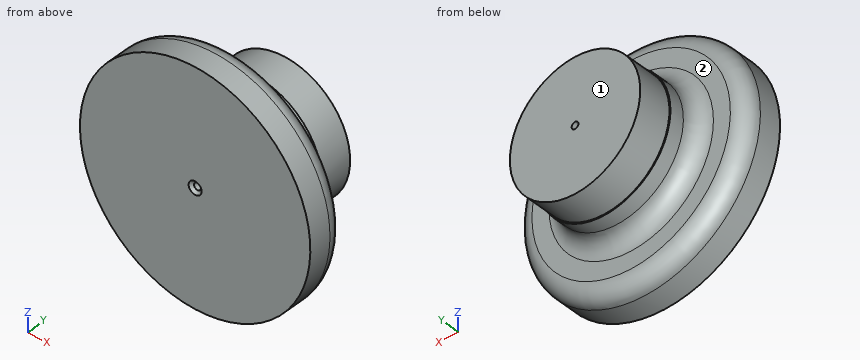
from build123d import *

# Parameters (mm, degrees)
SKETCH1_R                                           = 114.3
SKETCH1_R_2                                         = 65.7225
BOSS_EXTRUDE1_DEPTH                                 = 38.1
SKETCH1_3_R                                         = 65.7225
SKETCH1_3_R_2                                       = 64.7065
BOSS_EXTRUDE2_DEPTH                                 = 68.58
SKETCH1_4_R                                         = 64.7065
BOSS_EXTRUDE3_DEPTH                                 = 101.6
CSK_FOR_1_4_FLAT_HEAD_MACHINE_SCREW_100_D           = 6.7564
CSK_FOR_1_4_FLAT_HEAD_MACHINE_SCREW_100_CSINK_D     = 12.8778
CSK_FOR_1_4_FLAT_HEAD_MACHINE_SCREW_100_CSINK_ANGLE = 100
FILLET1_R                                           = 15.875
FILLET2_R                                           = 15.875


with BuildPart() as part:
    # Sketch1 → Boss-Extrude1 (new body)
    with BuildSketch(Plane(origin=(0, 0, 0), x_dir=(1, 0, 0), z_dir=(0, 1, 0))):
        with Locations(Location((0, 0, 0), (0, 0, 90))):
            Circle(SKETCH1_R)
        with Locations(Location((0, 0, 0), (0, 0, 90))):
            Circle(SKETCH1_R_2, mode=Mode.SUBTRACT)
    extrude(amount=BOSS_EXTRUDE1_DEPTH)

    # Sketch1_3 → Boss-Extrude2 (add)
    with BuildSketch(Plane(origin=(0, 0, 0), x_dir=(1, 0, 0), z_dir=(0, 1, 0))):
        with Locations(Location((0, 0, 0), (0, 0, 270))):
            Circle(SKETCH1_3_R)
        with Locations(Location((0, 0, 0), (0, 0, 270))):
            Circle(SKETCH1_3_R_2, mode=Mode.SUBTRACT)
    extrude(amount=BOSS_EXTRUDE2_DEPTH)

    # Sketch1_4 → Boss-Extrude3 (add)
    with BuildSketch(Plane(origin=(0, 0, 0), x_dir=(1, 0, 0), z_dir=(0, 1, 0))):
        with Locations(Location((0, 0, 0), (0, 0, 270))):
            Circle(SKETCH1_4_R)
    extrude(amount=BOSS_EXTRUDE3_DEPTH)

    # CSK for 1_4 Flat Head Machine Screw _100 (through all)
    with Locations(Plane(origin=(0, 0, 0), x_dir=(-1, 0, 0), z_dir=(0, -1, 0))):
        with Locations((0, 0)):
            CounterSinkHole(CSK_FOR_1_4_FLAT_HEAD_MACHINE_SCREW_100_D / 2, CSK_FOR_1_4_FLAT_HEAD_MACHINE_SCREW_100_CSINK_D / 2, counter_sink_angle=CSK_FOR_1_4_FLAT_HEAD_MACHINE_SCREW_100_CSINK_ANGLE)

    # Fillet1
    fillet1_edges = [part.edges().sort_by_distance(p)[0] for p in [
        (0, 38.1, -65.7225),
    ]]
    fillet(fillet1_edges, radius=FILLET1_R)

    # Fillet2
    fillet2_edges = [part.edges().sort_by_distance(p)[0] for p in [
        (0, 38.1, 114.3),
    ]]
    fillet(fillet2_edges, radius=FILLET2_R)


solid = part.part
Here's how the part is built. I have some questions about the finished solid (model axes, mm). Face numbers are marked on the shaded views. A direction names the side the tool comes from. Give positions to 0.01 mm unless a question says otherwise; leave off trailing zeros. Loops run counter-clockwise (first coordinate to the right, second up) from the corner with the lowest first, then second, coordinate; pieces in that order, holes last. Notation, with made-up numbers: (61, -1) -> (67, -1) arc R21 ccw to (67, 34) -> close; hole circle Ø3 at (-6.75, -0.5). An arc over 180 degrees is marked (long way). Answer as a JSON object with one key per item and string values. Group by question number.
Item 1: Imagine slicing it at C-C on y = 7.5. Write out the boundary of the cut face in (x, z), then the cut area to 3 significant figures.
Item 2: Imagine slicing it at D-D on y = 74. Write out the boundary of the cut face in (x, z).
Item 3: Will these pins go through, and if not, where does the flat tip stop? pin 1 (4 mm diameter, centred on x = 0, z = 0, fed in from -Y); pin 2 (5 mm diameter, centred on x = 3.5, y = 56, fed in from +Z); pin 3 (10 mm diameter, centred on y = 28.5, z = -1, fed in from -X); pin 4 (3 mm diameter, centred on x = -65, z = 72.5, fed in from +Y).
Item 4: On a 3-axis mill with a long thin cutter (end or side, diameter ignored), from which of +Z, -Z, +X, -X, +Y, -Y can I reach the whole of each face in a straight line? I mean the marked faces 1 and 2. Say none if no direction works.
Item 5: I need wall thicknesses on L1, parallel to Y at x = -65, z = 54; L2, parallel to X at y = 85, z = 58.5; L3, parallel to X at y = 6, z = 12.5. Which ranges of each line are inside material? Lowest first, please.
Answer list:
{
 "1": {"outline": "circle Ø228.6 at (0, 0); hole circle Ø6.76 at (0, 0)", "area": "41,000 mm2"},
 "2": {"outline": "circle Ø129.41 at (0, 0); hole circle Ø6.76 at (0, 0)"},
 "3": {"pin 1": "passes through", "pin 2": "stops at z = 65.71", "pin 3": "stops at x = -114.25", "pin 4": "stops at y = 38.1"},
 "4": {"face 1": "+Z, -Z, +X, -X, +Y", "face 2": "+Y"},
 "5": {"L1": "y = 0 to 38.1", "L2": "x = -27.65 to 27.65", "L3": "x = -113.61 to 113.61"}
}
